from build123d import *

# Parameters (mm, degrees)
SKETCH1_R           = 47.85
BOSS_EXTRUDE1_DEPTH = 222.25
SKETCH2_R           = 47.75
BOSS_EXTRUDE2_DEPTH = 57
FILLET1_R           = 47.85
SHELL1_T            = -5


with BuildPart() as part:
    # Sketch1 → Boss-Extrude1 (new body)
    with BuildSketch(Plane.XY):
        Circle(SKETCH1_R)
    extrude(amount=BOSS_EXTRUDE1_DEPTH)

    # Sketch2 → Boss-Extrude2 (add)
    with BuildSketch(Plane(origin=(0, 57, 0), x_dir=(1, 0, 0), z_dir=(0, 1, 0))):
        with Locations(Location((0, -60, 0), (0, 0, 270))):
            Circle(SKETCH2_R)
    extrude(amount=-BOSS_EXTRUDE2_DEPTH)

    # Sketch5 → Revolve3 (revolve)
    with BuildSketch(Plane(origin=(0, 0, 0), x_dir=(0, 0, -1), z_dir=(1, 0, 0)), mode=Mode.PRIVATE) as revolve3_sk:
        Polygon((-60, 57), (-12.25, 57), (-6.025, 63), (-6.025, 73.05), (-60, 73.05), align=None)
    revolve(revolve3_sk.sketch.rotate(Axis((0, 73.05, 60), (0, -1, 0)), 180), axis=Axis((0, 73.05, 60), (0, -1, 0)))

    # Fillet1
    fillet1_edges = [part.edges().sort_by_distance(p)[0] for p in [
        (-47.85, 0, 222.25),
    ]]
    fillet(fillet1_edges, radius=FILLET1_R)

    # Shell1
    shell1_openings = [part.faces().sort_by_distance(p)[0] for p in [
        (0, 73.05, 60),
        (0, 0, 0),
    ]]
    offset(amount=SHELL1_T, openings=shell1_openings, kind=Kind.INTERSECTION)


solid = part.part
Can you work these out from the model? Positions are in its coordinate system, mm. A direction names the side the tool comes from. Give positions to 0.01 mm unless a question says otherwise; leave off trailing zeros. Loops run counter-clockwise (first coordinate to the right, second up) from the corner with the lowest first, then second, coordinate; pieces in that order, holes last. Notation, with made-up numbers: M 74,-10.75 L 84,-10.75 A19 ccw 84,25.25 Z; hole C 87.25,26.5 d7. An arc over 180 degrees is marked long. One line per item, written item: value. Start each with the question number.
1) If we section it at C-C, the plane y = 0: Write out the boundary of the cut face in (x, z), and give its area (3 significant figures).
2) If I drill on line 1 (Y direction, x = 3, z = 129.5); line 2 (X direction, y = 35.5, z = 60); line 3 (X direction, y = 67, z = 60) (3 decimals), over which ranges is the centre line in solid material (lowest first)? Write a range as [from, to].
3) If we section it at B-B, the plane z = 60: Write out the boundary of the cut face in (x, y) (3 decimals).
4) If we section it at A-A, the plane x = 0: Write out the boundary of the cut face in (y, z) (3 decimals), and give its area (3 significant figures).
5) I'm going to push flat-ended pins straight in: pin 1 (5 mm diameter, centred on y = -34, z = 28.5, fed in from +X); pin 2 (12 mm diameter, centred on x = -35.5, y = 59.5, fed in from +Z); pin 3 (2 mm diameter, centred on x = 8.5, y = 43.5, fed in from +Z). Where does each tip first touch, or does it pass through?
6) On a 3-axis mill with a long thin cutter (end or side, diameter ignored), from which of +Z, -Z, +X, -X, +Y, -Y can I reach the whole of each face in a straight line? I mean faces 1 (the face through (-33.1, 69.143, 23.903)), 2 (the face through (-2.117, 57.375, 11.907)), 3 (the face through (-9.29, -41.83, 85.98)). Say none if no direction works.
7) Thinking about a two-plate mould opening in Y: for faces 4 (the face through (48, 73.05, 72)), 5 (the face through (-16.213, 68.095, 111.483)), 6 (the face through (-29.06, 42.4, 22.11)), which applies, +Y half, -Y half, draft (parallel to the pull), parting line (faces both ways), or undercut?
8) If we section it at D-D, the plane y = 54.5: Write out the boundary of the cut face in (x, z).
Completed:
1. outline: M -47.85,0 L -42.85,0 L -42.85,174.4 A42.85 cw 42.85,174.4 L 42.85,0 L 47.85,0 L 47.85,174.4 A47.85 ccw -47.85,174.4 Z
1. area: 2,460 mm^2
2. line 1: y = [-47.76, -42.74], [42.74, 47.76]
2. line 2: x = [-47.75, -42.75], [42.75, 47.75]
2. line 3: x = [-53.975, -48.975], [48.975, 53.975]
3. outline: M -53.975,63 L -47.75,57 L -47.75,3.092 A47.85 ccw long 47.75,3.092 L 47.75,57 L 53.975,63 L 53.975,73.05 L 48.975,73.05 L 48.975,65.125 L 42.75,59.125 L 42.75,2.926 A42.85 cw long -42.75,2.926 L -42.75,59.125 L -48.975,65.125 L -48.975,73.05 L -53.975,73.05 Z
4. outline: M -47.85,0 L -42.85,0 L -42.85,174.4 A42.85 cw 42.85,174.4 L 42.85,102.75 L 59.125,102.75 L 65.125,108.975 L 73.05,108.975 L 73.05,113.975 L 63,113.975 L 57,107.75 L 47.85,107.75 L 47.85,174.4 A47.85 ccw -47.85,174.4 Z; M 42.85,0 L 47.85,0 L 47.85,12.25 L 57,12.25 L 63,6.025 L 73.05,6.025 L 73.05,11.025 L 65.125,11.025 L 59.125,17.25 L 42.85,17.25 Z
4. area: 2,310 mm^2
5. pin 1: stops at x = 36.02
5. pin 2: stops at z = 104.44
5. pin 3: stops at z = 194.72
6. face 1: +Y
6. face 2: none
6. face 3: -Z
7. face 4: +Y half
7. face 5: draft
7. face 6: undercut
8. outline: C 0,60 d95.5; hole C 0,60 d85.5
